Source: CAD feature listing. Evaluate the final solid. Frame: model axes, mm. A direction names the side the tool comes from. Round coordinates to 2 decimals unless told otherwise and drop trailing zeros. Write each loop counter-clockwise with the first axis right and the second up, starting at its lowest first coordinate (ties: lowest second). Pieces come first, ordered by that corner, then holes.
```python
from build123d import *

# Parameters (mm, degrees)
BOSS_EXTRUDE1_DEPTH = 10
SKETCH2_R           = 8
SKETCH2_R_2         = 5.5
CUT_EXTRUDE2_DEPTH  = 4.3
SKETCH3_R           = 2.25
CUT_EXTRUDE3_DEPTH  = 22.656407828


with BuildPart() as part:
    # Sketch1 → Boss-Extrude1 (new body)
    with BuildSketch(Plane(origin=(0, 0, 0), x_dir=(0, 0, -1), z_dir=(1, 0, 0))):
        Polygon((-15, 0), (15, 0), (15, 8), (11, 12), (-11, 12), (-15, 8), align=None)
    extrude(amount=BOSS_EXTRUDE1_DEPTH)

    # Sketch2 → Cut-Extrude2 (cut)
    with BuildSketch(Plane(origin=(10, 0, 0), x_dir=(0, 0, -1), z_dir=(1, 0, 0))):
        with Locations((0, 3.5)):
            Circle(SKETCH2_R)
        with Locations((0, 3.5)):
            Circle(SKETCH2_R_2, mode=Mode.SUBTRACT)
    extrude(amount=-CUT_EXTRUDE2_DEPTH, mode=Mode.SUBTRACT)

    # Sketch3 → Cut-Extrude3 (cut, through all)
    with BuildSketch(Plane(origin=(10, 0, 0), x_dir=(0, 0, -1), z_dir=(1, 0, 0))):
        with Locations((-12, 4)):
            Circle(SKETCH3_R)
        with Locations((12, 4)):
            Circle(SKETCH3_R)
    extrude(amount=-CUT_EXTRUDE3_DEPTH, mode=Mode.SUBTRACT)


solid = part.part
```
Q1. Line query: line 1 (Y direction, x = 4.75, z = 12); line 2 (Z direction, x = 5, y = 2.75); line 3 (Y direction, x = 6, z = 0.25). Output: solid intervals per line, ascending.
Q2. Section query C-C, the plane y = 4. Output: boundary loops of the cut face in (x, z).
Q3. Mould query, pull axis Y, two halves, no side actions, for faces 3 (the face through (0, 6, 0)), 4 (the face through (5, 10, 13)), 5 (the face through (5, 0, 0)), 6 (the face through (5.7, 10, 0)). Classes: pulls with the +Y half, pulls with the -Y half, needs draft (parallel to the pull), parting line crosses it, or undercut.
Q4. Section query A-A, the plane z = 12. Output: boundary loops of the cut face in (x, y).
Q5. Section query B-B, the plane x = 4. Output: boundary loops of the cut face in (y, z), and give its area (3 significant figures).
Q6. Section query D-D, the plane x = 8.75. Output: boundary loops of the cut face in (y, z), and give its area (3 significant figures).
Q7. Pin query (flat end, axial travel): P1, Ø2, axis at x = 7, z = 7, coming from the -Y side; P2, Ø3, axis at x = 2.5, y = 10.5, coming from the +Z side. Return the tip coordinate at first contact, or that it passes through.
Q8. Set-up query: faces 1 (the face through (8, 9, 0)), 2 (the face through (5.07, 4.099, 14.248)). Return all of +Z, -Z, +X, -X, +Y, -Y with unobstructed straight access to the full face (end or side cutting, diameter ignored); none if empty.
Filled in:
1. line 1: y = 0 to 1.75, 6.25 to 11
1. line 2: z = -15 to -13.87, -10.13 to 10.13, 13.87 to 15
1. line 3: y = 0 to 8.99, 11.5 to 12
2. outline: (0, -15) - (10, -15) - (10, -14.25) - (0, -14.25) - close; (0, -9.75) - (10, -9.75) - (10, -7.98) - (5.7, -7.98) - (5.7, -5.48) - (10, -5.48) - (10, 5.48) - (5.7, 5.48) - (5.7, 7.98) - (10, 7.98) - (10, 9.75) - (0, 9.75) - close; (0, 14.25) - (10, 14.25) - (10, 15) - (0, 15) - close
3. face 3: needs draft
3. face 4: pulls with the +Y half
3. face 5: pulls with the -Y half
3. face 6: undercut
4. outline: (0, 0) - (10, 0) - (10, 1.75) - (0, 1.75) - close; (0, 6.25) - (10, 6.25) - (10, 11) - (0, 11) - close
5. outline: (0, -15) - (8, -15) - (12, -11) - (12, 11) - (8, 15) - (0, 15) - close; hole circle Ø4.5 at (4, -12); hole circle Ø4.5 at (4, 12)
5. area: 312 mm2
6. outline: (0, -15) - (8, -15) - (12, -11) - (12, 11) - (8, 15) - (0, 15) - (0, 7.19) arc R8 cw (long way) to (0, -7.19) - close; (0, -4.24) arc R5.5 ccw (long way) to (0, 4.24) - close; hole circle Ø4.5 at (4, -12); hole circle Ø4.5 at (4, 12)
6. area: 241 mm2
7. P1: stops at y = 0
7. P2: stops at z = 14
8. face 1: +X
8. face 2: +X, -X
